For this review, take the finished solid that the model builds, in its own axes (mm). A direction names the side the tool comes from. Coordinates: 2 decimals unless noted, no trailing zeros. Order: outer loops, then holes, each group sorted by start corner. A loop starts at its lowest first (then second) coordinate and runs counter-clockwise, first axis right, second up. Notation, with made-up numbers: (10, 71.25) -> (16, 71.25) arc R32 cw to (16, 107.25) -> close; hole circle Ø6 at (-34.5, -1). An arc over 180 degrees is marked (long way). Return JSON: item names as keys, results as strings. Group by question number.
Item 1: Machinability: for faces 1 (the flat face through (-1.95, 1.538, 12.32)), 2 (the cylindrical face through (-9.37, 0.27, 8.61)), 3 (the flat face through (8.4, 3, -8.4)), 4 (the flat face through (0, 10, 8)), 5 (the flat face through (4.2, 15, 0.2)), which of the approach directions +Z, -Z, +X, -X, +Y, -Y give a long, thin tool a straight path to every point of the face, cutting with its end or side? Answer none if there is none.
Item 2: Insertion check: pin 1 (4 mm diameter, centred on y = 4.5, z = 1.5, fed in from +X); pin 2 (5 mm diameter, centred on y = 13, z = -0.5, fed in from -X); pin 3 (3 mm diameter, centred on x = 0.5, z = -8, fed in from -Y). Each pin has a flat end and moves straight along its axis. Give the tip position at first contact, or say it passes through.
Item 3: For line 1 along Z through (x, y) = (0, 4.5); line 2 along Z through (x, y) = (0.5, 13.75); line 3 along Y through (x, z) = (-2.25, -8.75), list the stretches that pass through material, from the lowest coordinate up.
Item 4: Take a section at C-C (y = 12.5). Write out the cut boundary in (x, z).
Item 5: Take a section at A-A (y = 7.5). Write out the cut boundary in (x, z).
Item 6: Draft analysis for pull direction Y (two halves, no side actions). For faces 6 (the conical face through (-1.29, 14.87, 9.77)), 7 (the flat face through (1.93, 0.538, 12.32)), 8 (the cylindrical face through (-5.487, 4.93, -1.123)), state which applies: +Y half, -Y half, draft (parallel to the pull), parting line (faces both ways), or undercut.
Item 7: Take a section at B-B (y = 14). Write out the cut boundary in (x, z), then the cut area to 3 significant figures.
```python
from build123d import *

# Parameters (mm, degrees)
F0_R     = 11.7
F0_R_2   = 3
F0_R_3   = 4
F0_R_4   = 12.7
F1_DEPTH = 3
F2_DEPTH = 15
F3_DEPTH = 10
F7_SIZE  = 2


with BuildPart() as f1:
    # F0 (on Front) → F1 (new body)
    with BuildSketch(Plane.XZ):
        with Locations((-0.008065, 0.0265)):
            Circle(F0_R)
        with Locations((-0.008065, -8.2235)):
            Circle(F0_R_2, mode=Mode.SUBTRACT)
        with Locations((-8.258065, 0.0265)):
            Circle(F0_R_2, mode=Mode.SUBTRACT)
        with Locations((-0.008065, 0.0265)):
            Circle(F0_R_3, mode=Mode.SUBTRACT)
        with Locations((8.241935, 0.0265)):
            Circle(F0_R_2, mode=Mode.SUBTRACT)
        with Locations((-0.008065, 8.2765)):
            Circle(F0_R_2, mode=Mode.SUBTRACT)
        with Locations((-0.008065, 0.0265)):
            Circle(F0_R_4)
        with Locations((-0.008065, 0.0265)):
            Circle(F0_R, mode=Mode.SUBTRACT)
        with Locations((-8.258065, 0.0265)):
            Circle(F0_R_2)
        with Locations((-0.008065, -8.2235)):
            Circle(F0_R_2)
        with Locations((8.241935, 0.0265)):
            Circle(F0_R_2)
        with Locations((-0.008065, 8.2765)):
            Circle(F0_R_2)
    extrude(amount=-F1_DEPTH)

    # F0 (on Front) → F2 (join)
    with BuildSketch(Plane.XZ):
        with Locations((-0.008065, 0.0265)):
            Circle(F0_R)
        with Locations((-0.008065, -8.2235)):
            Circle(F0_R_2, mode=Mode.SUBTRACT)
        with Locations((-8.258065, 0.0265)):
            Circle(F0_R_2, mode=Mode.SUBTRACT)
        with Locations((-0.008065, 0.0265)):
            Circle(F0_R_3, mode=Mode.SUBTRACT)
        with Locations((8.241935, 0.0265)):
            Circle(F0_R_2, mode=Mode.SUBTRACT)
        with Locations((-0.008065, 8.2765)):
            Circle(F0_R_2, mode=Mode.SUBTRACT)
        with Locations((-8.258065, 0.0265)):
            Circle(F0_R_2)
        with Locations((-0.008065, 8.2765)):
            Circle(F0_R_2)
        with Locations((8.241935, 0.0265)):
            Circle(F0_R_2)
        with Locations((-0.008065, -8.2235)):
            Circle(F0_R_2)
    extrude(amount=-F2_DEPTH)

    # F0 (on Front) → F3 (cut)
    with BuildSketch(Plane.XZ):
        with Locations((-8.258065, 0.0265)):
            Circle(F0_R_2)
        with Locations((-0.008065, 8.2765)):
            Circle(F0_R_2)
        with Locations((8.241935, 0.0265)):
            Circle(F0_R_2)
        with Locations((-0.008065, -8.2235)):
            Circle(F0_R_2)
    extrude(amount=-F3_DEPTH, mode=Mode.SUBTRACT)

    # F4 (on Top) → F5 (revolve, cut)
    with BuildSketch(Plane.XY):
        with BuildLine():
            Line((-13.744461, 0.538489), (-12.316881, 0.538489))
            ThreePointArc((-12.316881, 0.538489), (-11.816881, 1.038489), (-12.316881, 1.538489))
            Line((-12.316881, 1.538489), (-12.716881, 1.538489))
            Line((-12.716881, 1.538489), (-13.744461, 1.538489))
            Line((-13.744461, 1.538489), (-13.744461, 0.538489))
        make_face()
    revolve(axis=Axis((0, 1.278264, 0), (0, 1, 0)), mode=Mode.SUBTRACT)

    # F4 (on Top) → F6 (revolve, cut)
    with BuildSketch(Plane.XY):
        with BuildLine():
            Line((-13.744461, 0.538489), (-12.316881, 0.538489))
            ThreePointArc((-12.316881, 0.538489), (-11.816881, 1.038489), (-12.316881, 1.538489))
            Line((-12.316881, 1.538489), (-12.716881, 1.538489))
            Line((-12.716881, 1.538489), (-13.744461, 1.538489))
            Line((-13.744461, 1.538489), (-13.744461, 0.538489))
        make_face()
    revolve(axis=Axis((0, 1.278264, 0), (0, 1, 0)), mode=Mode.SUBTRACT)

    # F7
    f7_edges = [f1.edges().sort_by_distance(p)[0] for p in [
        (-11.708065, 15, 0.0265),
    ]]
    chamfer(f7_edges, length=F7_SIZE)


solid = f1.part
```
Findings below:
{
 "1": {"face 1": "none", "face 2": "+Y, -Y", "face 3": "+Y", "face 4": "-Y", "face 5": "+Z, -Z, +X, -X, +Y"},
 "2": {"pin 1": "stops at x = 12.69", "pin 2": "stops at x = -11.71", "pin 3": "stops at y = 10"},
 "3": {"line 1": "z = -11.67 to -11.22, -5.22 to -3.97, 4.03 to 5.28, 11.28 to 11.73", "line 2": "z = -10.91 to -3.94, 3.99 to 10.96", "line 3": "y = 10 to 15"},
 "4": {"outline": "circle Ø23.4 at (-0.01, 0.03); hole circle Ø8 at (-0.01, 0.03)"},
 "5": {"outline": "circle Ø23.4 at (-0.01, 0.03); hole circle Ø6 at (-8.26, 0.03); hole circle Ø8 at (-0.01, 0.03); hole circle Ø6 at (-0.01, -8.22); hole circle Ø6 at (-0.01, 8.28); hole circle Ø6 at (8.24, 0.03)"},
 "6": {"face 6": "+Y half", "face 7": "undercut", "face 8": "draft"},
 "7": {"outline": "circle Ø21.4 at (-0.01, 0.03); hole circle Ø8 at (-0.01, 0.03)", "area": "309 mm2"}
}
